Geometry: see drawing. Coordinates: mm, zero at the bounding-box minimum. Coordinates: 2 decimals unless noted, no trailing zeros. Write each loop counter-clockwise with the first axis right and the second up, starting at its lowest first coordinate (ties: lowest second). Pieces come first, ordered by that corner, then holes. Notation, with made-up numbers: M 21,65.5 L 46,65.5 A30 ccw 46,103.5 Z; hole C 3.25,38.25 d6. An arc over 180 degrees is marked long. Write item = value, one per line. Start each with the question number.
1. Section query B-B (x = 587). Output: boundary loops of the cut face in (y, z).
2. Pin query (flat end, axial travel): pin 1 Ø8 at (x, y) = (617.5, 761.5) entering from -Z; pin 2 Ø12 at (y, z) = (688.5, 321) entering from -X; pin 3 Ø1 at (x, y) = (223, 388) entering from -Z. Return the tip coordinate at first contact, or that it passes through.
3. Section query A-A (y = 645.5). Output: boundary loops of the cut face in (x, z).
4. Section query C-C (z = 164). Output: boundary loops of the cut face in (x, y).
5. Section query D-D (y = 131). Output: boundary loops of the cut face in (x, z) (3 decimals).
6. Line query: line 1 along Y through (x, z) = (452, 521); line 2 along X through (y, z) = (634, 458.5); line 3 along X through (y, z) = (546, 404.5). Output: solid intervals per line, ascending.
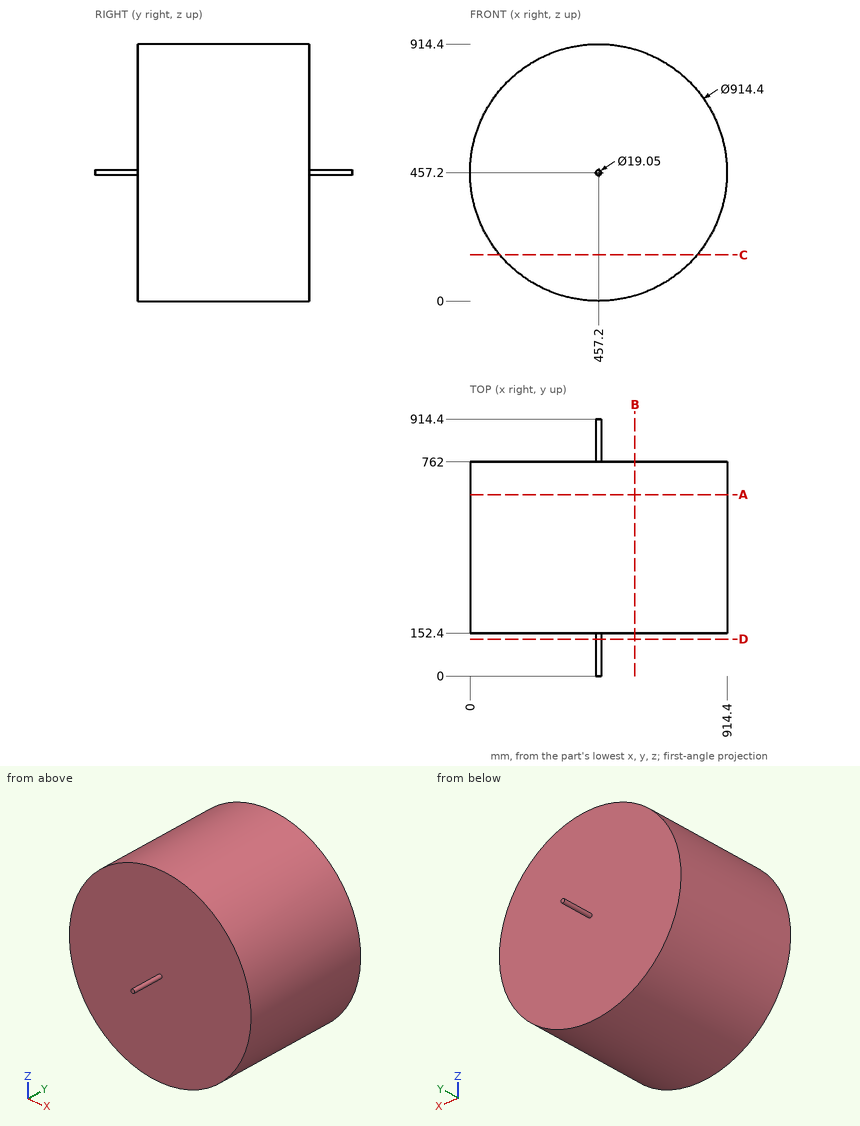
Results are:
q1.outline = M 152.4,18.81 L 762,18.81 L 762,895.59 L 152.4,895.59 Z
q2.pin_1 = 27.55
q2.pin_2 = 18.93
q2.pin_3 = 64.24
q3.outline = C 457.2,457.2 d914.4
q4.outline = M 106.39,152.4 L 808.01,152.4 L 808.01,762 L 106.39,762 Z
q5.outline = C 457.2,457.2 d19.05
q6.line_1 = 152.4 to 762
q6.line_2 = 0 to 914.4
q6.line_3 = 3.05 to 911.35
